Here's the drawing with two shaded views (mm, measured from the low corner). I have some questions. A direction names the side the tool comes from. Coordinates: 2 decimals unless noted, no trailing zeros. Write each loop counter-clockwise with the first axis right and the second up, starting at its lowest first coordinate (ties: lowest second). Pieces come first, ordered by that corner, then holes.
Item 1: If we section it at B-B (z = 10.25): Please give me the cut outline in (x, y) (3 decimals).
Item 2: If I drill on line 1 (Z direction, x = 6, y = 7.25); line 2 (Z direction, x = 55, y = 2.25); line 3 (X direction, y = 8.25, z = 15.25) (3 decimals), over which ranges is the centre line in solid material (lowest first)?
Item 3: I'm going to push a flat-ended pin straight in: pin 1 Ø10 at (x, z) = (22, 6) entering from -Y. Where does the tip first touch, or does it pass through?
Item 4: For the marked faces 1 and 2, which set-ups out of +Z, -Z, +X, -X, +Y, -Y let a thin tool reach every point of the face, with its end or its side?
Item 5: If we section it at A-A (y = 6.25): Please give me the cut outline in (x, z).
Item 6: If we section it at C-C (x = 55): Please give me the cut outline in (y, z) (3 decimals), then the cut area to 3 significant figures.
Item 7: If we section it at D-D (z = 15.25): Please give me the cut outline in (x, y) (3 decimals), then the cut area to 3 significant figures.
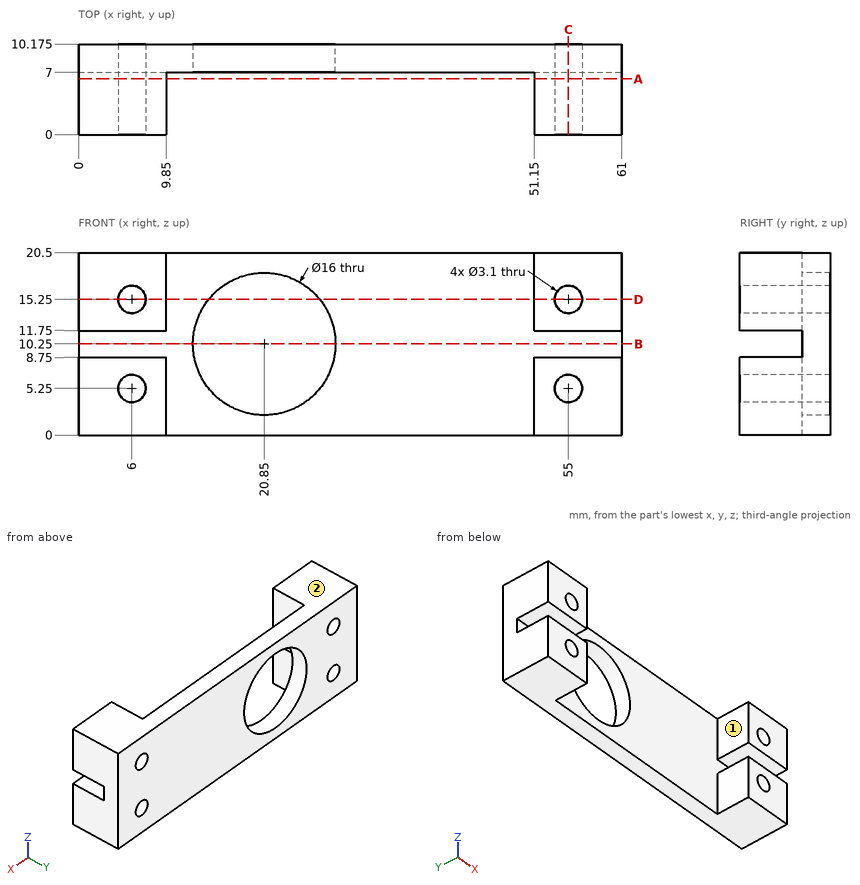
Answer list:
1. outline: (0, 7) - (12.85, 7) - (12.85, 10.175) - (0, 10.175) - close; (28.85, 7) - (61, 7) - (61, 10.175) - (28.85, 10.175) - close
2. line 1: z = 0 to 3.7, 6.8 to 13.7, 16.8 to 20.5
2. line 2: z = 0 to 3.7, 6.8 to 8.75, 11.75 to 13.7, 16.8 to 20.5
2. line 3: x = 0 to 4.45, 7.55 to 14.605, 27.095 to 53.45, 56.55 to 61
3. pin 1: stops at y = 7
4. face 1: +Z, -Z, -Y
4. face 2: +Z, +X, -X, +Y, -Y
5. outline: (0, 0) - (9.85, 0) - (9.85, 8.75) - (0, 8.75) - close; (0, 11.75) - (9.85, 11.75) - (9.85, 20.5) - (0, 20.5) - close; (51.15, 0) - (61, 0) - (61, 8.75) - (51.15, 8.75) - close; (51.15, 11.75) - (61, 11.75) - (61, 20.5) - (51.15, 20.5) - close; hole circle Ø3.1 at (6, 5.25); hole circle Ø3.1 at (6, 15.25); hole circle Ø3.1 at (55, 5.25); hole circle Ø3.1 at (55, 15.25)
6. outline: (0, 0) - (10.175, 0) - (10.175, 3.7) - (0, 3.7) - close; (0, 6.8) - (10.175, 6.8) - (10.175, 13.7) - (0, 13.7) - (0, 11.75) - (7, 11.75) - (7, 8.75) - (0, 8.75) - close; (0, 16.8) - (10.175, 16.8) - (10.175, 20.5) - (0, 20.5) - close
6. area: 125 mm2
7. outline: (0, 0) - (4.45, 0) - (4.45, 10.175) - (0, 10.175) - close; (7.55, 0) - (9.85, 0) - (9.85, 7) - (14.605, 7) - (14.605, 10.175) - (7.55, 10.175) - close; (27.095, 7) - (51.15, 7) - (51.15, 0) - (53.45, 0) - (53.45, 10.175) - (27.095, 10.175) - close; (56.55, 0) - (61, 0) - (61, 10.175) - (56.55, 10.175) - close
7. area: 229 mm2
